from build123d import *

# Parameters (mm, degrees)
SKETCH1_W           = 210.82
SKETCH1_H           = 210.82
BOSS_EXTRUDE1_DEPTH = 1.27
BOSS_EXTRUDE2_DEPTH = 17.78
SKETCH3_W           = 205.74
SKETCH3_H           = 205.74
SKETCH3_W_2         = 203.2
SKETCH3_H_2         = 203.2
BOSS_EXTRUDE3_DEPTH = 0.508
FILLET1_R           = 2.54
FILLET2_R           = 2.54


with BuildPart() as part:
    # Sketch1 → Boss-Extrude1 (new body)
    with BuildSketch(Plane(origin=(0, 0, 0), x_dir=(1, 0, 0), z_dir=(0, 1, 0))):
        Rectangle(SKETCH1_W, SKETCH1_H)
    extrude(amount=BOSS_EXTRUDE1_DEPTH)

    # Sketch2 → Boss-Extrude2 (add)
    with BuildSketch(Plane(origin=(0, 1.27, 0), x_dir=(1, 0, 0), z_dir=(0, 1, 0))):
        with BuildLine():
            Line((42.6085, -102.997), (42.6085, -104.14))
            ThreePointArc((42.6085, -104.14), (42.980474388, -105.038025612), (43.8785, -105.41))
            Line((43.8785, -105.41), (61.5315, -105.41))
            ThreePointArc((61.5315, -105.41), (62.429525612, -105.038025612), (62.8015, -104.14))
            Line((62.8015, -104.14), (62.8015, -102.997))
            ThreePointArc((62.8015, -102.997), (62.429525612, -102.098974388), (61.5315, -101.727))
            Line((61.5315, -101.727), (43.8785, -101.727))
            ThreePointArc((43.8785, -101.727), (42.980474388, -102.098974388), (42.6085, -102.997))
        make_face()
        with BuildLine():
            Line((-61.5315, -101.727), (-43.8785, -101.727))
            ThreePointArc((-43.8785, -101.727), (-42.980474388, -102.098974388), (-42.6085, -102.997))
            Line((-42.6085, -102.997), (-42.6085, -104.14))
            ThreePointArc((-42.6085, -104.14), (-42.980474388, -105.038025612), (-43.8785, -105.41))
            Line((-43.8785, -105.41), (-61.5315, -105.41))
            ThreePointArc((-61.5315, -105.41), (-62.429525612, -105.038025612), (-62.8015, -104.14))
            Line((-62.8015, -104.14), (-62.8015, -102.997))
            ThreePointArc((-62.8015, -102.997), (-62.429525612, -102.098974388), (-61.5315, -101.727))
        make_face()
    extrude(amount=BOSS_EXTRUDE2_DEPTH)

    # Sketch3 → Boss-Extrude3 (add)
    with BuildSketch(Plane.XZ):
        Rectangle(SKETCH3_W, SKETCH3_H)
        Rectangle(SKETCH3_W_2, SKETCH3_H_2, mode=Mode.SUBTRACT)
    extrude(amount=BOSS_EXTRUDE3_DEPTH)

    # Fillet1
    # the kernel refuses this fillet: 2.54 mm, written as the material it takes off along each edge
    with BuildSketch(Plane(origin=(105.41, 0, -110.909261314), x_dir=(0, 1, 0), z_dir=(0, 0, 1)), Plane(origin=(-110.909261314, 0, -105.41), x_dir=(0, 1, 0), z_dir=(1, 0, 0)), Plane(origin=(-105.41, 0, 110.909261314), x_dir=(0, 1, 0), z_dir=(0, 0, -1))) as fillet1_piece_1:
        with BuildLine():
            CenterArc((2.54, 2.199704526), FILLET1_R, 180, 60)
            Line((0, 2.199704526), (-0.0508, 2.199704526))
            Line((-0.0508, 2.199704526), (-0.0508, 0))
            Line((-0.0508, 0), (0, -0.0508))
            ThreePointArc((0, -0.0508), (0.635, -0.0508), (1.2446, -0.043994091))
            Line((1.2446, -0.043994091), (1.27, 0))
        make_face()
    extrude(amount=221.818522628, mode=Mode.SUBTRACT)

    # Fillet2
    # the kernel refuses this fillet: 2.54 mm, written as the material it takes off along each edge
    with BuildSketch(Plane(origin=(106.68, -0.508, 102.87), x_dir=(0, 1, 0), z_dir=(-1, 0, 0)), Plane(origin=(102.87, -0.508, -106.68), x_dir=(0, 1, 0), z_dir=(0, 0, 1)), Plane(origin=(-106.68, -0.508, -102.87), x_dir=(0, 1, 0), z_dir=(1, 0, 0)), Plane(origin=(-102.87, -0.508, 106.68), x_dir=(0, 1, 0), z_dir=(0, 0, -1))) as fillet2_piece_1:
        with BuildLine():
            CenterArc((2.54, 1.524), FILLET2_R, 180, 36.869897646)
            Line((0, 1.524), (-0.0508, 1.524))
            Line((-0.0508, 1.524), (-0.0508, 0))
            Line((-0.0508, 0), (0, -0.0508))
            ThreePointArc((0, -0.0508), (0.254, -0.0508), (0.46736, -0.03048))
            Line((0.46736, -0.03048), (0.508, 0))
        make_face()
    extrude(amount=213.36, mode=Mode.SUBTRACT)


solid = part.part
CAD build for the part. Positions are in the model's coordinates, mm. Give positions to 0.01 mm unless a question says otherwise; leave off trailing zeros. Order: outer loops, then holes, each group sorted by start corner. A loop starts at its lowest first (then second) coordinate and runs counter-clockwise, first axis right, second up. Notation, with made-up numbers: (69.5, 6.5) - (77.5, 6.5) arc R20 cw to (77.5, 34.5) - close; hole circle Ø3 at (11.5, 43). An arc over 180 degrees is marked (long way). Write each question's results on one line, items separated by ' | '.
1. Saw through at B-B on z = 33. List the corners of the cut face in (x, y), and give its area (3 significant figures).
Calculated:
outline: (-105.41, 1.27) arc R2.54 ccw to (-103.21, 0) - (-102.87, 0) arc R2.54 ccw to (-101.6, -0.5) - (-101.6, 0) - (101.6, 0) - (101.6, -0.5) arc R2.54 ccw to (102.87, 0) - (103.21, 0) arc R2.54 ccw to (105.41, 1.27) - close | area: 267 mm2
2. Pin check, flat tips, straight feed: pin 1 (1.3 mm diameter, centred on y = 12, z = 104, fed in from -X); pin 2 (0.9 mm diameter, centred on y = 6, z = 103.5, fed in from +X); pin 3 (4 mm diameter, centred on x = 0, z = 7, fed in from +Y); pin 4 (4 mm diameter, centred on x = -20, y = 2.5, fed in from +Z). Stop position of each tip, or through.
Calculated:
pin 1: stops at x = -62.8 | pin 2: stops at x = 62.8 | pin 3: stops at y = 1.27 | pin 4: stops at z = 105.41
3. Pull direction Z, two halves, no side cores. Call faces 1 (the face through (-0.5, 0.3, 105.41)), 2 (the face through (53, 10, 101.727)), 3 (the face through (-1, 0, -1)), 4 (the face through (-1, 1.27, -1)): released by +Z, released by -Z, zero draft, split by the parting line, or undercut.
Calculated:
face 1: released by +Z | face 2: released by -Z | face 3: undercut | face 4: zero draft
4. Saw through at D-D on x = -91. List the corners of the cut face in (y, z).
Calculated:
outline: (-0.5, -101.6) arc R2.54 ccw to (0, -102.87) - (0, -103.21) arc R2.54 ccw to (1.27, -105.41) - (1.27, 105.41) - (0, 105.41) - (0, 102.87) arc R2.54 ccw to (-0.5, 101.6) - (0, 101.6) - (0, -101.6) - close
5. Probe L1, parallel to Y at x = 43, z = -84; L2, parallel to Z at x = -55, y = 6.25. List the from-to ranges inside material, lowest first. Write a range as from..to.
Calculated:
L1: y = 0..1.27 | L2: z = 101.73..105.41
6. Saw through at A-A on y = 5. List the corners of the cut face in (x, z).
Calculated:
outline: (-62.8, 103) arc R1.27 ccw to (-61.53, 101.73) - (-43.88, 101.73) arc R1.27 ccw to (-42.61, 103) - (-42.61, 104.14) arc R1.27 ccw to (-43.88, 105.41) - (-61.53, 105.41) arc R1.27 ccw to (-62.8, 104.14) - close; (42.61, 103) arc R1.27 ccw to (43.88, 101.73) - (61.53, 101.73) arc R1.27 ccw to (62.8, 103) - (62.8, 104.14) arc R1.27 ccw to (61.53, 105.41) - (43.88, 105.41) arc R1.27 ccw to (42.61, 104.14) - close
7. Saw through at C-C on x = 57. List the corners of the cut face in (y, z).
Calculated:
outline: (-0.5, -101.6) arc R2.54 ccw to (0, -102.87) - (0, -103.21) arc R2.54 ccw to (1.27, -105.41) - (1.27, 101.73) - (19.05, 101.73) - (19.05, 105.41) - (0, 105.41) - (0, 102.87) arc R2.54 ccw to (-0.5, 101.6) - (0, 101.6) - (0, -101.6) - close
